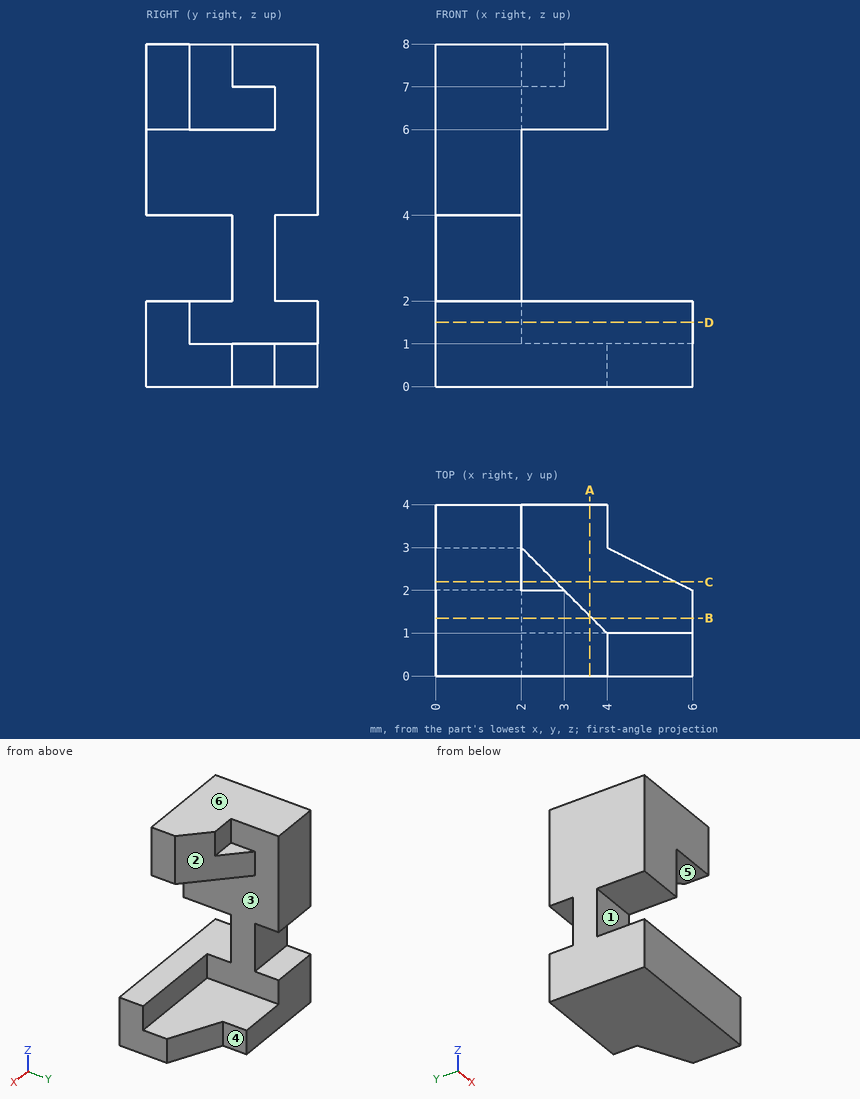
Verification items for this drawing (mm, ordinates from the low corner). A direction names the side the tool comes from. Round coordinates to 2 decimals unless told otherwise and drop trailing zeros. Loops run counter-clockwise (first coordinate to the right, second up) from the corner with the lowest first, then second, coordinate; pieces in that order, holes last. Notation, with made-up numbers: (-7.75, 35) -> (9.25, 35) arc R22 cw to (9.25, 71) -> close; hole circle Ø2 at (54, 86.5). An arc over 180 degrees is marked (long way). Write item = value, one per line. Start each with the question number.
1) Sectioned sample at C-C, the plane y = 2.2. Record the cut outline in (x, z).
2) Sectioned sample at A-A, the plane x = 3.6. Record the cut outline in (y, z), plus the area to 3 significant figures.
3) Sectioned sample at D-D, the plane z = 1.5. Record the cut outline in (x, y), plus the area to 3 significant figures.
4) Sectioned sample at B-B, the plane y = 1.35. Record the cut outline in (x, z), plus the area to 3 significant figures.
5) Thickness scan on probe 1 along Z at (x, y) = (1.45, 3.4); probe 2 along Z at (x, y) = (3.5, 2); probe 3 along X at (y, z) = (2.6, 4). Record the ranges inside material, lowest first.
6) Set-up check for the marked faces 1, 2 and 3: record each of +Z, -Z, +X, -X, +Y, -Y from which the full face is reachable in a straight line by a thin tool's end or side.
7) Release check for a two-part mould opening along Z. For the marked faces 4, 5 and 6 record: released by +Z, released by -Z, zero draft, split by the parting line, or undercut.
8) Gauge pin test, flat ends, axial feed: pin 1 Ø0.5 at (x, y) = (1, 3.5) entering from -Z; pin 2 Ø0.5 at (y, z) = (3.5, 0.5) entering from +X; pin 3 Ø0.5 at (x, y) = (2.5, 2.5) entering from +Z; pin 4 Ø0.6 at (x, y) = (4.5, 0.5) entering from +Z. Record the tip position at first contact, or that the pin passes through.
Results are:
q1.outline = (0, 0) -> (5.6, 0) -> (5.6, 1) -> (2, 1) -> (2, 6) -> (2.8, 6) -> (2.8, 7) -> (2, 7) -> (2, 8) -> (0, 8) -> close
q2.outline = (0, 0) -> (4, 0) -> (4, 1) -> (1, 1) -> (1, 2) -> (0, 2) -> close; (0, 6) -> (1.4, 6) -> (1.4, 8) -> (0, 8) -> close
q2.area = 7.80 mm^2
q3.outline = (0, 0) -> (6, 0) -> (6, 1) -> (2, 1) -> (2, 4) -> (0, 4) -> close
q3.area = 12.0 mm^2
q4.outline = (0, 0) -> (6, 0) -> (6, 1) -> (2, 1) -> (2, 2) -> (0, 2) -> close; (0, 4) -> (2, 4) -> (2, 6) -> (3.65, 6) -> (3.65, 8) -> (0, 8) -> close
q4.area = 19.3 mm^2
q5.probe_1 = 0 to 2, 4 to 8
q5.probe_2 = 0 to 1
q5.probe_3 = 0 to 2
q6.face_1 = +X, -X, -Y
q6.face_2 = +Z, +X, +Y
q6.face_3 = +X, +Y
q7.face_4 = zero draft
q7.face_5 = undercut
q7.face_6 = released by +Z
q8.pin_1 = 0
q8.pin_2 = 4
q8.pin_3 = 7
q8.pin_4 = 2
